Geometry check sheet. Reference: the model listing, model coordinates, mm. A direction names the side the tool comes from. Give positions to 0.01 mm unless a question says otherwise; leave off trailing zeros. Loops run counter-clockwise (first coordinate to the right, second up) from the corner with the lowest first, then second, coordinate; pieces in that order, holes last.
1. Cross-section at B-B, the plane x = 12.5. Record the cut outline in (y, z), plus the area to 3 significant figures.
2. Cross-section at D-D, the plane x = 32. Record the cut outline in (y, z), plus the area to 3 significant figures.
3. Material ranges on L1, parallel to X at y = 2.95, z = 0; L2, parallel to Z at x = 12.5, y = 2.85; L3, parallel to Z at x = 16.5, y = 0.8, recorded low to high.
4. Go/stop test with flat-tipped pins: pin 1 Ø1.2 at (x, y) = (34, 2.5) entering from +Z; pin 2 Ø2 at (x, y) = (37.5, 1.5) entering from -Z; pin 3 Ø1.2 at (y, z) = (2.5, -32) entering from +X. Record where each tip stops, or that it passes through.
5. Cross-section at C-C, the plane y = 1.5. Record the cut outline in (x, z), plus the area to 3 significant figures.
6. Cross-section at A-A, the plane z = 0. Record the cut outline in (x, y), plus the area to 3 significant figures.
7. Tool access check on faces 4 (the flat face through (35, 2, 0)), 5 (the flat face through (-37, 2, -20)), 6 (the flat face through (-30, 2, -30)), 7 (the flat face through (30, 2, -30)). Record the directions out of +Z, -Z, +X, -X, +Y, -Y that give a thin tool (end or side, any length) a straight path to the whole face; none if there is none.
8. Release check for a two-part mould opening along Z. For faces 1 (the flat face through (-39, 2, 25)), 2 (the flat face through (0, 2, 34)), 3 (the cylindrical face through (0.012, 2.028, -0.55)) record: +Z half, -Z half, draft (parallel to the pull), parting line (faces both ways), or undercut.
Autodesk Inventor part; units mm, degrees
ref_plane "YZ Plane" through (0, 0, 0) normal (1, 0, 0) x (0, 1, 0)
ref_plane "XZ Plane" through (0, 0, 0) normal (0, 1, 0) x (-1, 0, 0)
ref_plane "XY Plane" through (0, 0, 0) normal (0, 0, 1) x (1, 0, 0)
sketch "Sketch1" plane through (0, 0, 0) normal (0, 1, 0) x (-1, 0, 0)
  line L0 (35, 30) -> (-35, 30) construction
  line L1 (-35, 30) -> (-35, -30) construction
  line L2 (-35, -30) -> (35, -30) construction
  line L3 (35, -30) -> (35, 30) construction
  line L4 (-35, -20) -> (-39, -20)
  line L5 (-39, -20) -> (-39, -30)
  line L6 (-39, -30) -> (-35, -30)
  line L7 (-35, -30) -> (-35, -20) construction
  line L8 (-35, 20) -> (-39, 20)
  line L9 (-39, 20) -> (-39, 30)
  line L10 (-39, 30) -> (-35, 30)
  line L11 (-35, 30) -> (-35, 20) construction
  line L12 (35, 30) -> (39, 30)
  line L13 (39, 30) -> (39, 20)
  line L14 (39, 20) -> (35, 20)
  line L15 (35, 20) -> (35, 30) construction
  line L16 (35, -30) -> (39, -30)
  line L17 (39, -30) -> (39, -20)
  line L18 (39, -20) -> (35, -20)
  line L19 (35, -20) -> (35, -30) construction
  line L20 (20, -30) -> (35, -30) construction
  line L21 (35, -30) -> (35, -34) construction
  line L22 (35, -34) -> (20, -34) construction
  line L23 (20, -34) -> (20, -30)
  line L24 (-20, -30) -> (-35, -30) construction
  line L25 (-35, -30) -> (-35, -34) construction
  line L26 (-35, -34) -> (-20, -34) construction
  line L27 (-20, -34) -> (-20, -30)
  line L28 (-35, 30) -> (-20, 30)
  line L29 (-20, 30) -> (-20, 34)
  line L30 (-20, 34) -> (-35, 34) construction
  line L31 (-35, 34) -> (-35, 30) construction
  line L32 (20, 34) -> (35, 34) construction
  line L33 (35, 34) -> (35, 30) construction
  line L34 (35, 30) -> (20, 30)
  line L35 (20, 30) -> (20, 34)
  line L36 (20, -30) -> (-20, -30) construction
  line L37 (-35, 20) -> (-35, -20)
  line L38 (35, -20) -> (35, 20)
  line L39 (20, 30) -> (-20, 30) construction
  line L40 (35, -30) -> (20, -30)
  line L41 (20, -34) -> (-20, -34)
  line L42 (-20, -30) -> (-35, -30)
  line L43 (-20, 34) -> (20, 34)
  line L44 (20, 30) -> (35, 30)
  point P0 (0, 0)
  point P1 (37, 20)
  point P2 (37, -20)
  point P3 (-20, -32)
  point P4 (20, -32)
  point P5 (0, -30)
  point P6 (35, 0)
  dimension "d0" = 70
  dimension "d1" = 60
  dimension "d2" = 4
  dimension "d3" = 40
  dimension "d4" = 40
extrude "Extrusion1" add sketch "Sketch1" along normal blind 4
sketch "Sketch2" plane through (0, 4, 0) normal (0, 1, 0) x (1, 0, 0)
  circle A0 centre (12.5, 0) radius 12.5
  line L0 (35, -20) -> (35, 20)
  point P0 (0, 0)
  dimension "d7" = 25
  dimension "d8" = 10
extrude "Extrusion2" cut sketch "Sketch2" against normal blind 4
properties part number "SideFemale_70wx60h" material "Wood (Oak)"
Result:
1. outline: (0, -34) - (4, -34) - (4, -12.5) - (0, -12.5) - close; (0, 12.5) - (4, 12.5) - (4, 34) - (0, 34) - close
1. area: 172 mm2
2. outline: (0, -30) - (4, -30) - (4, 30) - (0, 30) - close
2. area: 240 mm2
3. L1: x = -35 to 0, 25 to 35
3. L2: z = -34 to -12.5, 12.5 to 34
3. L3: z = -34 to -11.84, 11.84 to 34
4. pin 1: stops at z = 30
4. pin 2: stops at z = -30
4. pin 3: stops at x = 20
5. outline: (-39, -30) - (-20, -30) - (-20, -34) - (20, -34) - (20, -30) - (39, -30) - (39, -20) - (35, -20) - (35, 20) - (39, 20) - (39, 30) - (20, 30) - (20, 34) - (-20, 34) - (-20, 30) - (-39, 30) - (-39, 20) - (-35, 20) - (-35, -20) - (-39, -20) - close; hole circle Ø25 at (12.5, 0)
5. area: 4,190 mm2
6. outline: (-35, 0) - (0, 0) - (0, 4) - (-35, 4) - close; (25, 0) - (35, 0) - (35, 4) - (25, 4) - close
6. area: 180 mm2
7. face 4: +X, +Y, -Y
7. face 5: -X, +Y, -Y
7. face 6: -Z, -X, +Y, -Y
7. face 7: -Z, +X, +Y, -Y
8. face 1: draft
8. face 2: +Z half
8. face 3: undercut
